Could you check a few things on this model? Use its own coordinates, in mm. Coordinates: 2 decimals unless noted, no trailing zeros. Write each loop counter-clockwise with the first axis right and the second up, starting at its lowest first coordinate (ties: lowest second). Pieces come first, ordered by that corner, then holes.
Autodesk Inventor part; units mm, degrees
ref_plane "YZ Plane" through (0, 0, 0) normal (1, 0, 0) x (0, 1, 0)
ref_plane "XZ Plane" through (0, 0, 0) normal (0, 1, 0) x (-1, 0, 0)
ref_plane "XY Plane" through (0, 0, 0) normal (0, 0, 1) x (1, 0, 0)
sketch "Szkic1" plane through (0, 0, 0) normal (0, 1, 0) x (-1, 0, 0)
  circle A0 centre (0, 0) radius 1.5
  line L0 (-2, 2) -> (2, 2)
  line L1 (2, 2) -> (2, -2)
  line L2 (2, -2) -> (-2, -2)
  line L3 (-2, -2) -> (-2, 2)
  line L4 (-2, 2) -> (2, -2) construction
  line L5 (2, 2) -> (-2, -2) construction
  line L6 (0, 0) -> (0, -23)
  line L7 (0, 0) -> (23, 0) construction
  line L8 (2, 2) -> (-2, 2)
  line L9 (-2, 2) -> (-2, -22)
  line L10 (-2, -22) -> (2, -22)
  line L11 (2, -22) -> (2, 2)
  circle A1 centre (0, -44) radius 1.5
  line L12 (-2, -46) -> (2, -46)
  line L13 (2, -46) -> (2, -42)
  line L14 (2, -42) -> (-2, -42)
  line L15 (-2, -42) -> (-2, -46)
  line L16 (-2, -46) -> (2, -42) construction
  line L17 (2, -46) -> (-2, -42) construction
  line L18 (0, -44) -> (0, -23)
  line L19 (0, -44) -> (23, -44) construction
  line L20 (2, -46) -> (-2, -46)
  line L21 (-2, -46) -> (-2, -22)
  line L22 (2, -22) -> (2, -46)
  dimension "d0" = 3
  dimension "d1" = 4
  dimension "d2" = 4
  dimension "d3" = 23
  dimension "d4" = 90
  dimension "d5" = 4
  dimension "d6" = 24
extrude "Wyciągnięcie proste1" add sketch "Szkic1" along normal blind 6.8
fillet "Zaokrąglenie1" radius 2 4 edges at (-2, 3.4, 2) (2, 3.4, 2) (-2, 3.4, -46) (2, 3.4, -46)
sketch "Szkic2" plane through (0, 6.8, 0) normal (0, 1, 0) x (1, 0, 0)
  circle A0 centre (0, 0) radius 1.5
  circle A1 centre (0, 0) radius 1.5
  circle A2 centre (0, 0) radius 2
extrude "Wyciągnięcie proste2" add sketch "Szkic2" along normal blind 3.5
properties part number "link_sub"
Item 1: I want a section at A-A, the plane y = 6. Count the separate pieces of the cut face and the enclosed holes in it, then the cut area to 3 significant figures.
Item 2: If I drill on line 1 along Z through (x, y) = (0, 3.75); line 2 along X through (y, z) = (4.75, 0); line 3 along Z through (x, y) = (-0.55, 3.25), over which ranges is the centre line in solid material (lowest first)?
Item 3: Will these pins go through, and if not, where does the flat tip stop? pin 1 Ø1.8 at (x, z) = (0, 0) entering from +Y; pin 2 Ø2 at (x, z) = (1, -7) entering from -Y.
Item 4: I want a section at B-B, the plane z = -26.5. List the corners of the cut face in (x, y) for me.
Item 5: If we mould it in two halves opening along Z, with no side actions, what happens to faces 1 (the cylindrical face through (0.325, 3.352, -42.536)), 2 (the cylindrical face through (-1.4, 3.45, -45.43)), 3 (the cylindrical face through (1.848, 8.526, -0.766))? For each: released by +Z, released by -Z, zero draft, split by the parting line, or undercut.
Taken from the geometry:
1. separate pieces: 1
1. enclosed holes: 2
1. area: 174 mm2
2. line 1: z = -46 to -45.5, -42.5 to -1.5, 1.5 to 2
2. line 2: x = -2 to -1.5, 1.5 to 2
2. line 3: z = -45.92 to -45.4, -42.6 to -1.4, 1.4 to 1.92
3. pin 1: passes through
3. pin 2: stops at y = 0
4. outline: (-2, 0) - (2, 0) - (2, 6.8) - (-2, 6.8) - close
5. face 1: undercut
5. face 2: released by -Z
5. face 3: split by the parting line
